Study the drawing (mm; zero at the part's minimum x, y, z) and answer. Give positions to 0.01 mm unless a question says otherwise; leave off trailing zeros. Order: outer loops, then holes, each group sorted by start corner. A loop starts at its lowest first (then second) coordinate and runs counter-clockwise, first axis right, second up. Notation, with made-up numbers: (64.5, 8) - (91.5, 8) arc R19 ccw to (91.5, 31) - close; hole circle Ø11 at (13.25, 64). An arc over 180 degrees is marked (long way). Write each question's results on one line, items separated by ' | '. Start each with the question number.
Q1. Find section A-A on y = 0.9. Give the vertices of the cut face in (x, z).
Q2. Find the intervals of material crossed by line 1 along X through (y, z) = (1.1, 20); line 2 along Y through (x, z) = (2.5, 18), in increasing order. Write a range as from..to.
Q3. Find section D-D on x = 1.2. Give the vertices of the cut face in (y, z).
Q4. For a pull along X with two mould halves and no side action, classify the marked faces 1, 2 and 3 as +X half, -X half, draft (parallel to the pull), parting line (faces both ways), or undercut.
Q5. Find section B-B on z = 15. Give the vertices of the cut face in (x, y).
Q6. A flat-ended cylindrical pin translates along its axis: P1, Ø0.6, axis at x = 4, y = 0, coming from the +Z side. Find the tip coordinate at first contact, or state that the pin passes through.
Q7. Find section C-C on x = 3.45. Give the vertices of the cut face in (y, z).
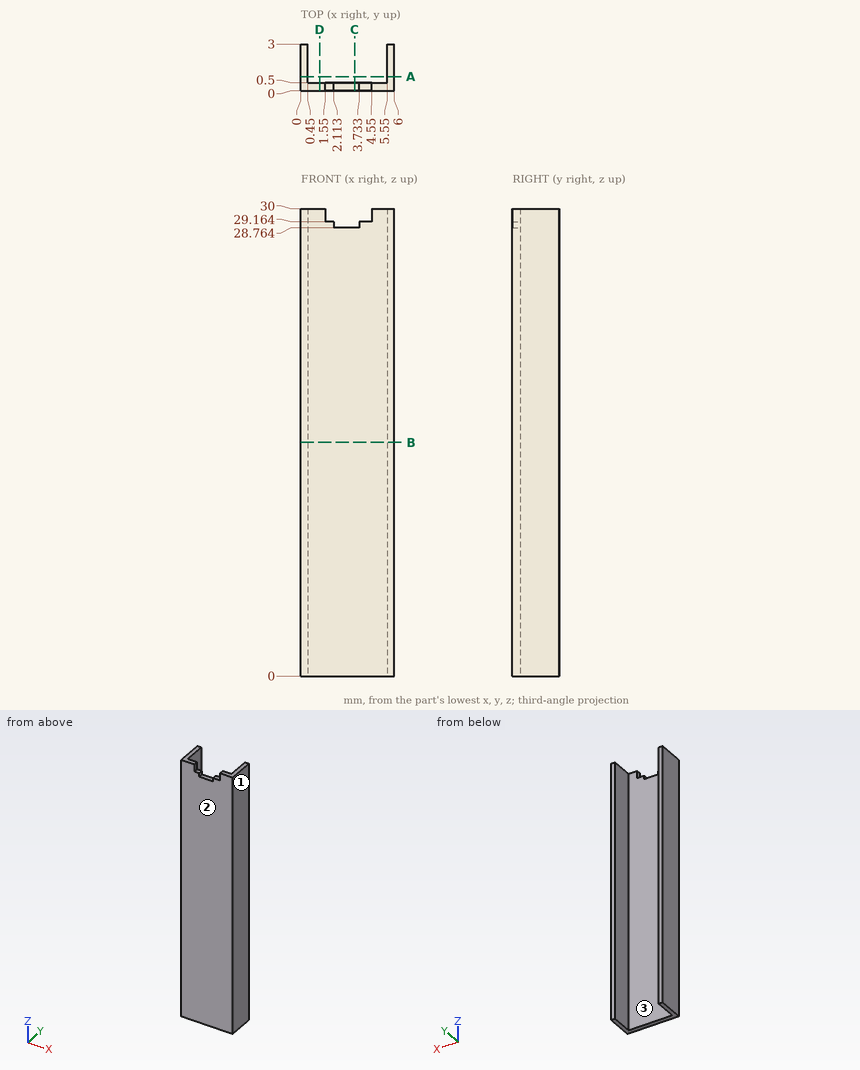
Working result:
1) outline: (0, 0) - (0.45, 0) - (0.45, 30) - (0, 30) - close; (5.55, 0) - (6, 0) - (6, 30) - (5.55, 30) - close
2) line 1: 0..0.45, 5.55..6 | line 2: 0..0.5
3) outline: (0, 0) - (0.5, 0) - (0.5, 30) - (0, 30) - close
4) face 1: +X half | face 2: draft | face 3: undercut
5) outline: (0, 0) - (6, 0) - (6, 3) - (5.55, 3) - (5.55, 0.5) - (0.45, 0.5) - (0.45, 3) - (0, 3) - close
6) P1: z = 29.16
7) outline: (0, 0) - (0.5, 0) - (0.5, 28.76) - (0, 28.76) - close
